Here's how the part is built. I have some questions about the finished solid (model axes, mm). A direction names the side the tool comes from. Coordinates: 2 decimals unless noted, no trailing zeros. Write each loop counter-clockwise with the first axis right and the second up, starting at its lowest first coordinate (ties: lowest second). Pieces come first, ordered by that corner, then holes.
```python
from build123d import *

# Parameters (mm, degrees)
SKETCH1_W           = 66.04
SKETCH1_H           = 58.135485311
SKETCH1_R           = 1.5875
BOSS_EXTRUDE1_DEPTH = 3.175


with BuildPart() as part:
    # Sketch1 → Boss-Extrude1 (new body)
    with BuildSketch(Plane(origin=(0, 0, 0), x_dir=(1, 0, 0), z_dir=(0, 1, 0))):
        with Locations((0, -4.325528995)):
            Rectangle(SKETCH1_W, SKETCH1_H)
        with Locations(Location((29.845, 21.56721366, 0), (0, 0, 90))):
            Circle(SKETCH1_R, mode=Mode.SUBTRACT)
        with Locations(Location((29.845, -30.218271651, 0), (0, 0, 270))):
            Circle(SKETCH1_R, mode=Mode.SUBTRACT)
        with Locations(Location((-29.845, -30.218271651, 0), (0, 0, 90))):
            Circle(SKETCH1_R, mode=Mode.SUBTRACT)
        with Locations(Location((-29.845, 21.56721366, 0), (0, 0, 270))):
            Circle(SKETCH1_R, mode=Mode.SUBTRACT)
        Polygon((-26.67, -23.573367042), (-4.805088789, -4.325528996), (-26.67, 14.92230905), align=None, mode=Mode.SUBTRACT)
        Polygon((-21.00151998, 18.39221366), (0, -0.095574897), (21.00151998, 18.39221366), align=None, mode=Mode.SUBTRACT)
        Polygon((0, -8.555483095), (21.00151998, -27.043271651), (-21.00151998, -27.043271651), align=None, mode=Mode.SUBTRACT)
        Polygon((4.805088789, -4.325528996), (26.67, 14.92230905), (26.67, -23.573367042), align=None, mode=Mode.SUBTRACT)
    extrude(amount=BOSS_EXTRUDE1_DEPTH)


solid = part.part
```
1) Imagine slicing it at A-A on z = 7.5. Please give me the cut outline in (x, y) (3 decimals), then the cut area to 3 significant figures.
Values follow:
outline: (-33.02, 0) - (-26.67, 0) - (-26.67, 3.175) - (-33.02, 3.175) - close; (-8.411, 0) - (8.411, 0) - (8.411, 3.175) - (-8.411, 3.175) - close; (26.67, 0) - (33.02, 0) - (33.02, 3.175) - (26.67, 3.175) - close
area: 93.7 mm2
2) I need wall thicknesses on probe 1 along X at (y, z) = (2.6, -21.5); probe 2 along Z at (x, y) = (0, 1.65); probe 3 along X at (y, z) = (1.05, 5.5). Which ranges of each line are inside material? Lowest first, please.
Values follow:
probe 1: x = -33.02 to -31.43, -28.26 to 28.26, 31.43 to 33.02
probe 2: z = -24.74 to -18.39, 0.1 to 8.56, 27.04 to 33.39
probe 3: x = -33.02 to -26.67, -6.14 to 6.14, 26.67 to 33.02
3) Imagine slicing it at D-D on x = -23.5. Please give me the cut outline in (y, z) (3 decimals), then the cut area to 3 significant figures.
Values follow:
outline: (0, -24.742) - (3.175, -24.742) - (3.175, -12.132) - (0, -12.132) - close; (0, 20.783) - (3.175, 20.783) - (3.175, 33.393) - (0, 33.393) - close
area: 80.1 mm2
4) On a 3-axis mill with a long thin cutter (end or side, diameter ignored), from which of +Z, -Z, +X, -X, +Y, -Y can I reach the whole of each face in a straight line? I mean faces 1 (the face through (0, 2, -18.392)), 2 (the face through (0, 2, -24.742)). Say none if no direction works.
Values follow:
face 1: +Y, -Y
face 2: -Z, +X, -X, +Y, -Y
5) Imagine slicing it at C-C on z = -5. Please give me the cut outline in (x, y) (3 decimals).
Values follow:
outline: (-33.02, 0) - (-26.67, 0) - (-26.67, 3.175) - (-33.02, 3.175) - close; (-15.399, 0) - (-5.788, 0) - (-5.788, 3.175) - (-15.399, 3.175) - close; (5.788, 0) - (15.399, 0) - (15.399, 3.175) - (5.788, 3.175) - close; (26.67, 0) - (33.02, 0) - (33.02, 3.175) - (26.67, 3.175) - close
6) We'd pull the mould along Z, two halves only. Please class faces 3 (the face through (-28.295, 1.565, 30.562)), 4 (the face through (-10.65, 1.57, -9.28)), 5 (the face through (0, 0, 4)), 6 (the face through (0, 2, 33.393)): pulls with the +Z half, pulls with the -Z half, needs draft (parallel to the pull), parting line crosses it, or undercut.
Values follow:
face 3: undercut
face 4: undercut
face 5: needs draft
face 6: pulls with the +Z half
7) Imagine slicing it at B-B on x = 29. Please give me the cut outline in (y, z) (3 decimals), then the cut area to 3 significant figures.
Values follow:
outline: (0, -24.742) - (3.175, -24.742) - (3.175, -22.911) - (0, -22.911) - close; (0, -20.223) - (3.175, -20.223) - (3.175, 28.874) - (0, 28.874) - close; (0, 31.562) - (3.175, 31.562) - (3.175, 33.393) - (0, 33.393) - close
area: 168 mm2
